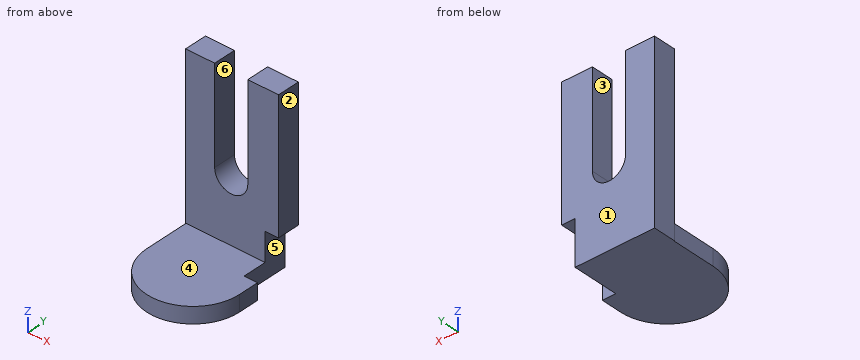
```python
from build123d import *

# Parameters (mm, degrees)
F0_W     = 54.2243942618
F0_H     = 102.3101732135
F1_DEPTH = 13.208
F2_W     = 19.3572593853
F2_H     = 55.7058900595
F3_DEPTH = 42.164
F6_W     = 54.037803784
F6_H     = 39.4023768604
F7_DEPTH = 9.398
F4_W     = 15.2707248926
F4_H     = 29.6811275184
F8_DEPTH = 27.178


with BuildPart() as f1:
    # F0 (on Front) → F1 (new body)
    with BuildSketch(Plane.XZ):
        with Locations((-0.0431220978, 4.4882334769)):
            Rectangle(F0_W, F0_H)
    extrude(amount=F1_DEPTH)

    # F2 (on Front) → F3 (cut)
    with BuildSketch(Plane.XZ):
        with Locations((-0.5377004854, 27.8529450297)):
            Rectangle(F2_W, F2_H)
        with BuildLine():
            Line((9.1409292072, 0), (-10.2163301781, 0))
            ThreePointArc((-10.2163301781, 0), (-0.5377004854, -9.6786296926), (9.1409292072, 0))
        make_face()
    extrude(amount=F3_DEPTH, mode=Mode.SUBTRACT)

    # F6 (on offset) → F7 (join)
    with BuildSketch(Plane(origin=(0, 0, -46.6668531299), x_dir=(1, 0, 0), z_dir=(0, 0, -1))):
        with Locations((0.077442266, 19.7011884302)):
            Rectangle(F6_W, F6_H)
        with BuildLine():
            ThreePointArc((27.0963441581, 39.4023768604), (0.077442266, 66.4212787524), (-26.941459626, 39.4023768604))
            Line((-26.941459626, 39.4023768604), (27.0963441581, 39.4023768604))
        make_face()
    extrude(amount=-F7_DEPTH)

    # F4 (on Front) → F8 (cut)
    with BuildSketch(Plane.XZ):
        with Locations((26.8850810826, -35.4883056134)):
            Rectangle(F4_W, F4_H)
    extrude(amount=F8_DEPTH, mode=Mode.SUBTRACT)


solid = f1.part
```
Verification items for the finished model (mm, model axes). Face numbers are marked on the shaded views. A direction names the side the tool comes from. Give positions to 0.01 mm unless a question says otherwise; leave off trailing zeros. Write each loop counter-clockwise with the first axis right and the second up, starting at its lowest first coordinate (ties: lowest second). Pieces come first, ordered by that corner, then holes. Notation, with made-up numbers: M 69,76 L 85,76 A17 cw 85,94 Z; hole C 22.25,10.5 d3. An arc over 180 degrees is marked long. One line per question, with ' | ' between items.
1) Mould release check, pull along X, two halves, no side actions. Record for the marked faces 1, 2 and 3: released by +X, released by -X, zero draft, split by the parting line, or undercut.
Result:
face 1: zero draft | face 2: released by +X | face 3: undercut
2) Gauge pin test, flat ends, axial feed: pin 1 Ø3 at (x, y) = (-11.5, -50.5) entering from +Z; pin 2 Ø12 at (x, z) = (12, -4) entering from +Y; pin 3 Ø8.5 at (x, y) = (25, -3.5) entering from -Z; pin 4 Ø3 at (y, z) = (-28.5, -41) entering from -X. Record the tip position at first contact, or that the pin passes through.
Result:
pin 1: stops at z = -37.27 | pin 2: stops at y = 0 | pin 3: stops at z = -20.65 | pin 4: stops at x = -26.94
3) Section check D-D on y = -25. Enter the section's corners in (x, z), plus the area to 3 significant figures.
Result:
outline: M -26.94,-46.67 L 19.25,-46.67 L 19.25,-37.27 L -26.94,-37.27 Z | area: 434 mm2
4) Set-up check for the marked faces 4, 5 and 6: record each of +Z, -Z, +X, -X, +Y, -Y from which the full face is reachable in a straight line by a thin tool's end or side.
Result:
face 4: +Z, +X, -X, -Y | face 5: -Z, +X, +Y | face 6: +Z, +Y, -Y
5) Section check B-B on x = -22. Enter the section's corners in (y, z).
Result:
outline: M -54.98,-46.67 L 0,-46.67 L 0,55.64 L -13.21,55.64 L -13.21,-37.27 L -54.98,-37.27 Z
6) Section check C-C on z = -25.5. Enter the section's corners in (x, y), plus the area to 3 significant figures.
Result:
outline: M -27.16,-13.21 L 19.25,-13.21 L 19.25,0 L -27.16,0 Z | area: 613 mm2
7) Section check A-A on z = 31. Enter the section's corners in (x, y), plus the area to 3 significant figures.
Result:
outline: M -27.16,-13.21 L -10.22,-13.21 L -10.22,0 L -27.16,0 Z; M 9.14,-13.21 L 27.07,-13.21 L 27.07,0 L 9.14,0 Z | area: 461 mm2
8) Thickness scan on line 1 along Z through (x, y) = (9, -18); line 2 along X through (y, z) = (-11, -26); line 3 along Y through (x, z) = (-16.5, 45.5). Record the ranges inside material, lowest first. Write a range as [from, to].
Result:
line 1: z = [-46.67, -37.27] | line 2: x = [-27.16, 19.25] | line 3: y = [-13.21, 0]
